Geometry check sheet. Reference: the model listing, model coordinates, mm. A direction names the side the tool comes from. Give positions to 0.01 mm unless a question says otherwise; leave off trailing zeros. Order: outer loops, then holes, each group sorted by start corner. A loop starts at its lowest first (then second) coordinate and runs counter-clockwise, first axis right, second up. Notation, with made-up numbers: (65, 32.5) - (108, 32.5) arc R26 cw to (108, 52.5) - close; hole circle Ø6 at (79, -38). An arc over 180 degrees is marked (long way). Put each result on its own line as item: value. Start each with the question number.
```python
from build123d import *

# Parameters (mm, degrees)
SKETCH1_W                                           = 101.6
SKETCH1_H                                           = 101.6
BOSS_EXTRUDE1_DEPTH                                 = 3.175
SKETCH19_W                                          = 12.75921203
SKETCH19_H                                          = 12.60998148
SKETCH19_W_2                                        = 12.60998148
SKETCH19_H_2                                        = 12.75921203
CUT_EXTRUDE1_DEPTH                                  = 3.175
F_3_4_0_75_DIAMETER_HOLE1_D                         = 19.05
SKETCH29_W                                          = 71.12
SKETCH29_H                                          = 6.858
BOSS_EXTRUDE11_DEPTH                                = 3.048
SKETCH30_W                                          = 7.950155684
SKETCH30_H                                          = 6.858
SKETCH30_W_2                                        = 7.931445158
BOSS_EXTRUDE12_DEPTH                                = 149.352
SKETCH31_W                                          = 4.703535678
SKETCH31_H                                          = 6.858
BOSS_EXTRUDE13_DEPTH                                = 55.88
SKETCH32_W                                          = 18.396349522
SKETCH32_H                                          = 14.53383174
SKETCH32_W_2                                        = 18.288
SKETCH32_H_2                                        = 14.533831847
SKETCH32_W_3                                        = 18.317097516
SKETCH32_H_3                                        = 14.559025954
BOSS_EXTRUDE14_DEPTH                                = 2.032
CBORE_FOR_2_BINDING_HEAD_MACHINE_SCREW1_D           = 2.4384
CBORE_FOR_2_BINDING_HEAD_MACHINE_SCREW1_CBORE_D     = 5.55752
CBORE_FOR_2_BINDING_HEAD_MACHINE_SCREW1_CBORE_DEPTH = 1.27


with BuildPart() as part:
    # Sketch1 → Boss-Extrude1 (new body)
    with BuildSketch(Plane.XY):
        with Locations((52.482861157, 13.097719286)):
            Rectangle(SKETCH1_W, SKETCH1_H)
    extrude(amount=BOSS_EXTRUDE1_DEPTH)

    # Sketch19 → Cut-Extrude1 (cut)
    with BuildSketch(Plane.XY.offset(3.175)):
        with Locations((11.237467172, 54.417728546)):
            Rectangle(SKETCH19_W, SKETCH19_H)
        with Locations((93.802870417, -28.147674699)):
            Rectangle(SKETCH19_W_2, SKETCH19_H_2)
        with Locations((93.802870417, 54.417728546)):
            Rectangle(SKETCH19_W_2, SKETCH19_H)
        with Locations((11.237467172, -28.147674699)):
            Rectangle(SKETCH19_W, SKETCH19_H_2)
    extrude(amount=-CUT_EXTRUDE1_DEPTH, mode=Mode.SUBTRACT)

    # 3/4 (0.75) Diameter Hole1 (through all)
    with Locations(Plane(origin=(0, 0, 0), x_dir=(-1, 0, 0), z_dir=(0, 0, -1))):
        with Locations((-52.482861157, 13.097719286)):
            Hole(F_3_4_0_75_DIAMETER_HOLE1_D / 2)

    # Sketch29 → Boss-Extrude11 (add)
    with BuildSketch(Plane.XY.offset(3.175)):
        with Locations((52.482988157, 41.418719286)):
            Rectangle(SKETCH29_W, SKETCH29_H)
    extrude(amount=BOSS_EXTRUDE11_DEPTH)

    # Sketch30 → Boss-Extrude12 (add)
    with BuildSketch(Plane.XY.offset(6.223)):
        with Locations((84.067910315, 41.418719286)):
            Rectangle(SKETCH30_W, SKETCH30_H)
        with Locations((20.888710736, 41.418719286)):
            Rectangle(SKETCH30_W_2, SKETCH30_H)
    extrude(amount=BOSS_EXTRUDE12_DEPTH)

    # Sketch31 → Boss-Extrude13 (add)
    with BuildSketch(Plane.ZY.offset(-80.092832473)):
        with Locations((153.223232161, 41.418719286)):
            Rectangle(SKETCH31_W, SKETCH31_H)
    extrude(amount=BOSS_EXTRUDE13_DEPTH)

    # Sketch32 → Boss-Extrude14 (add)
    with BuildSketch(Plane(origin=(0, 44.847719286, 0), x_dir=(1, 0, 0), z_dir=(0, 1, 0))):
        with Locations((76.304813396, -148.30808413)):
            Rectangle(SKETCH32_W, SKETCH32_H)
        with Locations((28.606988157, -148.30808413)):
            Rectangle(SKETCH32_W_2, SKETCH32_H)
        with Locations((76.304813396, -10.441915924)):
            Rectangle(SKETCH32_W, SKETCH32_H_2)
        with Locations((28.621536915, -10.454512977)):
            Rectangle(SKETCH32_W_3, SKETCH32_H_3)
    extrude(amount=BOSS_EXTRUDE14_DEPTH)

    # CBORE for #2 Binding Head Machine Screw1 (through all)
    with Locations(Plane(origin=(0, 46.879719286, 0), x_dir=(1, 0, 0), z_dir=(0, 1, 0))):
        with Locations((31.071863114, -12.257454761), (72.45160574, -12.257454761), (72.45160574, -146.811730834), (31.071863114, -146.811730834)):
            CounterBoreHole(CBORE_FOR_2_BINDING_HEAD_MACHINE_SCREW1_D / 2, CBORE_FOR_2_BINDING_HEAD_MACHINE_SCREW1_CBORE_D / 2, CBORE_FOR_2_BINDING_HEAD_MACHINE_SCREW1_CBORE_DEPTH)


solid = part.part
```
Item 1: Gauge pin test, flat ends, axial feed: pin 1 Ø2 at (y, z) = (45.5, 13.5) entering from +X; pin 2 Ø2 at (y, z) = (46.5, 149.5) entering from -X; pin 3 Ø2 at (y, z) = (42, 55) entering from -X; pin 4 Ø2 at (x, z) = (72.45, 146.81) entering from -Y. Record the tip position at first contact, or that the pin passes through.
Item 2: Cross-section at B-B (x = 45). Enter the section's corners in (y, z) (3 decimals).
Item 3: Thickness scan on line 1 along X through (y, z) = (44, 104); line 2 along Z through (x, y) = (41, 43) (3 decimals); line 3 along Y through (x, z) = (86, 50). Record the ranges inside material, lowest first.
Item 4: Cross-section at C-C (y = 10). Enter the section's corners in (x, z) (3 decimals), and give its area (3 significant figures).
Item 5: Cross-section at A-A (z = 24.5). Enter the section's corners in (x, y), and give its area (3 significant figures).
Item 6: Cross-section at D-D (x = 8). Enter the section's corners in (y, z) (3 decimals), and give its area (3 significant figures).
Item 7: Set-up check for faces 3 (the face through (53, 44.848, 153)), 4 (the face through (53, 41, 150.871)), 5 (the face through (74, 45.61, 13)): record each of +Z, -Z, +X, -X, +Y, -Y from which the full face is reachable in a straight line by a thin tool's end or side.
Item 8: Release check for a two-part mould opening along Z. For faces 1 (the face through (31, 44.848, 145)), 2 (the face through (50.42, 3.8, 1.61)) record: +Z half, -Z half, draft (parallel to the pull), parting line (faces both ways), or undercut.
Recorded:
1. pin 1: stops at x = 88.04
1. pin 2: stops at x = 19.46
1. pin 3: stops at x = 16.92
1. pin 4: passes through
2. outline: (-37.702, 0) - (7.204, 0) - (7.204, 3.175) - (-37.702, 3.175) - close; (18.991, 0) - (63.898, 0) - (63.898, 3.175) - (44.848, 3.175) - (44.848, 6.223) - (37.99, 6.223) - (37.99, 3.175) - (18.991, 3.175) - close; (37.99, 150.871) - (44.848, 150.871) - (44.848, 155.575) - (37.99, 155.575) - close
3. line 1: x = 16.92 to 24.85, 80.09 to 88.04
3. line 2: z = 0 to 6.223, 150.871 to 155.575
3. line 3: y = 37.99 to 44.85
4. outline: (1.683, 0) - (43.476, 0) - (43.476, 3.175) - (1.683, 3.175) - close; (61.49, 0) - (103.283, 0) - (103.283, 3.175) - (61.49, 3.175) - close
4. area: 265 mm^2
5. outline: (16.92, 37.99) - (24.85, 37.99) - (24.85, 44.85) - (16.92, 44.85) - close; (80.09, 37.99) - (88.04, 37.99) - (88.04, 44.85) - (80.09, 44.85) - close
5. area: 109 mm^2
6. outline: (-37.702, 0) - (-34.527, 0) - (-34.527, 3.175) - (-37.702, 3.175) - close; (-21.768, 0) - (48.113, 0) - (48.113, 3.175) - (-21.768, 3.175) - close; (60.723, 0) - (63.898, 0) - (63.898, 3.175) - (60.723, 3.175) - close
6. area: 242 mm^2
7. face 3: +Z, +Y
7. face 4: -Y
7. face 5: +Y
8. face 1: undercut
8. face 2: draft
